```python
from build123d import *

# Parameters (mm, degrees)
SKETCH1_R           = 1.75
SKETCH1_W           = 16
SKETCH1_H           = 5.5
BOSS_EXTRUDE1_DEPTH = 3


with BuildPart() as part:
    # Sketch1 → Boss-Extrude1 (new body)
    # profile 1 of 2: a face of its own
    with BuildSketch(Plane.XY):
        with BuildLine():
            Line((-3, 18.5), (3, 18.5))
            ThreePointArc((3, 18.5), (5.121320344, 17.621320344), (6, 15.5))
            Line((6, 15.5), (6, -15.5))
            Line((6, -15.5), (-6, -15.5))
            Line((-6, -15.5), (-6, 15.5))
            ThreePointArc((-6, 15.5), (-5.121320344, 17.621320344), (-3, 18.5))
        make_face()
        with Locations((0, 12.5)):
            Circle(SKETCH1_R, mode=Mode.SUBTRACT)
        with BuildLine():
            Line((1.75, -3), (1.75, -6))
            ThreePointArc((1.75, -6), (0, -7.75), (-1.75, -6))
            Line((-1.75, -6), (-1.75, -3))
            ThreePointArc((-1.75, -3), (0, -1.25), (1.75, -3))
        make_face(mode=Mode.SUBTRACT)
    # profile 2 of 2: a face of its own
    with BuildSketch(Plane.XY):
        with Locations((0, -12.75)):
            Rectangle(SKETCH1_W, SKETCH1_H)
    extrude(amount=BOSS_EXTRUDE1_DEPTH)


solid = part.part
```
Verification items for the finished model (mm, model axes). A direction names the side the tool comes from. Coordinates: 2 decimals unless noted, no trailing zeros. Loops run counter-clockwise (first coordinate to the right, second up) from the corner with the lowest first, then second, coordinate; pieces in that order, holes last. Notation, with made-up numbers: (48, -12) - (70, -12) arc R11 ccw to (70, -4) - close; hole circle Ø9 at (4, 39). An arc over 180 degrees is marked (long way). Return JSON: item names as keys, results as strings.
1. Mould release check, pull along Y, two halves, no side actions. Record for faces 5 (the flat face through (-1.75, -5, 1)), 6 (the flat face through (7, -10, 1)), 7 (the flat face through (-6, 3, 1)): +Y half, -Y half, draft (parallel to the pull), parting line (faces both ways), or undercut.
Established:
{"face 5": "undercut", "face 6": "+Y half", "face 7": "draft"}
2. Section check A-A, the plane y = 12.5. Record the boundary of the cut face in (x, z).
Established:
{"outline": "(-6, 0) - (-1.75, 0) - (-1.75, 3) - (-6, 3) - close; (1.75, 0) - (6, 0) - (6, 3) - (1.75, 3) - close"}
3. Section check B-B, the plane z = 1.15. Record the boundary of the cut face in (x, y), then the cut area to 3 significant figures.
Established:
{"outline": "(-8, -15.5) - (8, -15.5) - (8, -10) - (6, -10) - (6, 15.5) arc R3 ccw to (3, 18.5) - (-3, 18.5) arc R3 ccw to (-6, 15.5) - (-6, -10) - (-8, -10) - close; hole (-1.75, -6) arc R1.75 ccw to (1.75, -6) - (1.75, -3) arc R1.75 ccw to (-1.75, -3) - close; hole circle Ø3.5 at (0, 12.5)", "area": "396 mm2"}
4. Thickness scan on L1, parallel to Y at x = 0, z = 1.7; L2, parallel to Y at x = 1.5, z = 2.3; L3, parallel to X at y = -3.5, z = 1. Record the ranges inside material, lowest first.
Established:
{"L1": "y = -15.5 to -7.75, -1.25 to 10.75, 14.25 to 18.5", "L2": "y = -15.5 to -6.9, -2.1 to 11.6, 13.4 to 18.5", "L3": "x = -6 to -1.75, 1.75 to 6"}
5. Section check D-D, the plane y = 8. Record the boundary of the cut face in (x, z).
Established:
{"outline": "(-6, 0) - (6, 0) - (6, 3) - (-6, 3) - close"}
6. Tool access check on faces 1 (the flat face through (8, -13, 1)), 2 (the flat face through (6, 3, 1)), 3 (the flat face through (-7, -10, 1)), 4 (the flat face through (1.75, -4, 1)). Record the directions out of +Z, -Z, +X, -X, +Y, -Y that give a thin tool (end or side, any length) a straight path to the whole face; none if there is none.
Established:
{"face 1": "+Z, -Z, +X, +Y, -Y", "face 2": "+Z, -Z, +X, +Y", "face 3": "+Z, -Z, -X, +Y", "face 4": "+Z, -Z"}
7. Go/stop test with flat-tipped pins: pin 1 (1 mm diameter, centred on x = 7, z = 1, fed in from +Y); pin 2 (1 mm diameter, centred on y = 13.5, z = 1.5, fed in from +X); pin 3 (1.5 mm diameter, centred on y = -5, z = 1, fed in from -X). Record where each tip stops, or that it passes through.
Established:
{"pin 1": "stops at y = -10", "pin 2": "stops at x = 6", "pin 3": "stops at x = -6"}
8. Section check C-C, the plane x = 0.5. Record the boundary of the cut face in (y, z).
Established:
{"outline": "(-15.5, 0) - (-7.68, 0) - (-7.68, 3) - (-15.5, 3) - close; (-1.32, 0) - (10.82, 0) - (10.82, 3) - (-1.32, 3) - close; (14.18, 0) - (18.5, 0) - (18.5, 3) - (14.18, 3) - close"}
